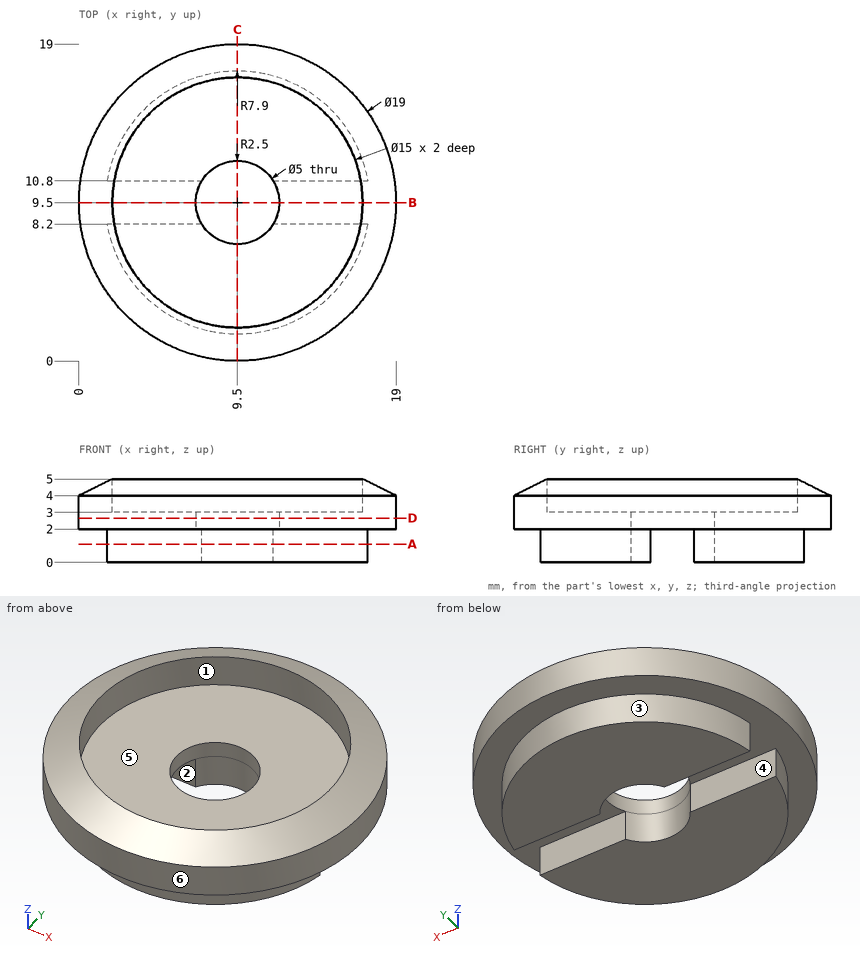
The drawing under review shows one solid part. Ordinate dimensions are in mm from its lowest x, y, z. A direction names the side the tool comes from. Give positions to 0.01 mm unless a question says otherwise; leave off trailing zeros. Order: outer loops, then holes, each group sorted by start corner. A loop starts at its lowest first (then second) coordinate and runs counter-clockwise, first axis right, second up. Notation, with made-up numbers: (-6, -3.75) -> (16, -3.75) arc R8 ccw to (16, 8.25) -> close; hole circle Ø10 at (-25.75, -5). An arc over 180 degrees is marked (long way). Write item = value, one per line.
1) We need section B-B, the plane y = 9.5. Give the boundary of the cut face in (x, z), and give its area (3 significant figures).
Findings:
outline = (0, 2) -> (7, 2) -> (7, 3) -> (2, 3) -> (2, 5) -> (0, 4) -> close; (12, 2) -> (19, 2) -> (19, 4) -> (17, 5) -> (17, 3) -> (12, 3) -> close
area = 20.0 mm^2
2) We need section D-D, the plane z = 2.65. Give the boundary of the cut face in (x, y), and give its area (3 significant figures).
Findings:
outline = circle Ø19 at (9.5, 9.5); hole circle Ø5 at (9.5, 9.5)
area = 264 mm^2
3) We need section C-C, the plane x = 9.5. Give the boundary of the cut face in (y, z), and give its area (3 significant figures).
Findings:
outline = (0, 2) -> (1.6, 2) -> (1.6, 0) -> (7, 0) -> (7, 3) -> (2, 3) -> (2, 5) -> (0, 4) -> close; (12, 0) -> (17.4, 0) -> (17.4, 2) -> (19, 2) -> (19, 4) -> (17, 5) -> (17, 3) -> (12, 3) -> close
area = 41.6 mm^2
4) Insertion check: pin 1 (0.6 mm diameter, centred on x = 15, z = 1, fed in from +Y); pin 2 (1 mm diameter, centred on x = 4.5, z = 2, fed in from +Y); pin 3 (2 mm diameter, centred on x = 14.5, y = 3.5, fed in from +Z); pin 4 (0.6 mm diameter, centred on x = 4.5, z = 1, fed in from -Y). Each pin has a flat end and moves straight along its axis. Give the tip position at first contact, or say it passes through.
Findings:
pin_1 = 15.45
pin_2 = 17.87
pin_3 = 5
pin_4 = 3.15
5) We need section A-A, the plane z = 1.1. Give the boundary of the cut face in (x, y).
Findings:
outline = (1.71, 8.2) arc R7.9 ccw to (17.29, 8.2) -> (11.64, 8.2) arc R2.5 cw to (7.36, 8.2) -> close; (1.71, 10.8) -> (7.36, 10.8) arc R2.5 cw to (11.64, 10.8) -> (17.29, 10.8) arc R7.9 ccw to start
6) To check wall thickness, follow L1, parallel to Y at x = 9.5, z = 2.4; L2, parallel to Y at x = 9.5, z = 3.55. State the ranges of each line that lie inside material, in increasing order. Write a range as from..to.
Findings:
L1 = 0..7, 12..19
L2 = 0..2, 17..19
7) For the marked faces 4, 5 and 6, list the 3-axis set-ups (+Z, -Z, +X, -X, +Y, -Y) from which the entire face can be reached by the end or side of a thin tool; tool diameter is ignored.
Findings:
face_4 = -Z, +X, -X
face_5 = +Z
face_6 = +Z, -Z
8) Draft analysis for pull direction X (two halves, no side actions). For the marked faces 1, 2 and 3, state which applies: pulls with the +X half, pulls with the -X half, needs draft (parallel to the pull), parting line crosses it, or undercut.
Findings:
face_1 = undercut
face_2 = needs draft
face_3 = parting line crosses it
